from build123d import *

# Parameters (mm, degrees)
SKETCH1_W           = 355.6
SKETCH1_H           = 203.2
SKETCH1_R           = 2.413
BOSS_EXTRUDE1_DEPTH = 3.175
SKETCH2_R           = 3.81
CUT_EXTRUDE1_DEPTH  = 205.80595847


with BuildPart() as part:
    # Sketch1 → Boss-Extrude1 (new body)
    with BuildSketch(Plane(origin=(0, 0, 0), x_dir=(1, 0, 0), z_dir=(0, 1, 0))):
        Rectangle(SKETCH1_W, SKETCH1_H)
        with Locations(Location((42.8625, 74.240027739, 0), (0, 0, 270))):
            Circle(SKETCH1_R, mode=Mode.SUBTRACT)
        with Locations(Location((85.725, 0, 0), (0, 0, 270))):
            Circle(SKETCH1_R, mode=Mode.SUBTRACT)
        with Locations(Location((42.8625, -74.240027739, 0), (0, 0, 270))):
            Circle(SKETCH1_R, mode=Mode.SUBTRACT)
        with Locations(Location((-42.8625, -74.240027739, 0), (0, 0, 270))):
            Circle(SKETCH1_R, mode=Mode.SUBTRACT)
        with Locations(Location((-85.725, 0, 0), (0, 0, 270))):
            Circle(SKETCH1_R, mode=Mode.SUBTRACT)
        with Locations(Location((-42.8625, 74.240027739, 0), (0, 0, 270))):
            Circle(SKETCH1_R, mode=Mode.SUBTRACT)
    extrude(amount=BOSS_EXTRUDE1_DEPTH)

    # Sketch2 → Cut-Extrude1 (cut, through all)
    with BuildSketch(Plane(origin=(0, 3.175, 0), x_dir=(1, 0, 0), z_dir=(0, 1, 0))):
        with Locations(Location((165.1, 82.55, 0), (0, 0, 270))):
            Circle(SKETCH2_R)
        with Locations(Location((-165.1, 82.55, 0), (0, 0, 90))):
            Circle(SKETCH2_R)
        with Locations(Location((-165.1, -82.55, 0), (0, 0, 270))):
            Circle(SKETCH2_R)
        with Locations(Location((165.1, -82.55, 0), (0, 0, 90))):
            Circle(SKETCH2_R)
    extrude(amount=-CUT_EXTRUDE1_DEPTH, mode=Mode.SUBTRACT)


solid = part.part
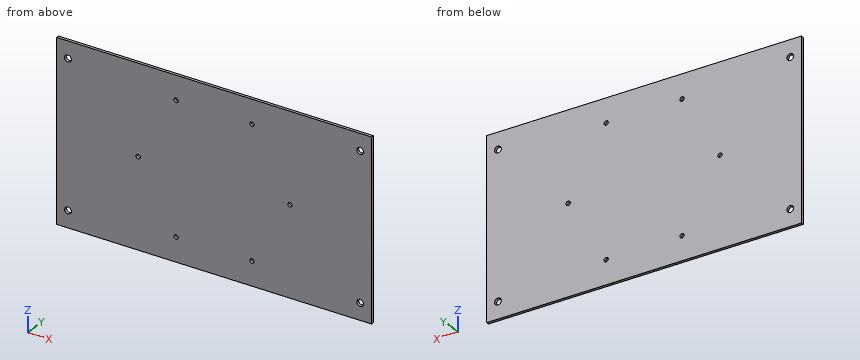
Read the model definition and answer for the solid it produces. Units are mm, in the model's axes. Give positions to 0.01 mm unless a question says otherwise; leave off trailing zeros. Write each loop counter-clockwise with the first axis right and the second up, starting at its lowest first coordinate (ties: lowest second). Pieces come first, ordered by that corner, then holes. Notation, with made-up numbers: (-30, -6) - (-25, -6) arc R23 ccw to (-25, 13) - close; hole circle Ø6 at (54.5, 11). An arc over 180 degrees is marked (long way). Return JSON: item names as keys, results as strings.
Q1. A cutting plane is placed at B-B, the plane z = 82.55. Determine the outline of the cut face in (x, y) (3 decimals).
Reply:
{"outline": "(-177.8, 0) - (-168.91, 0) - (-168.91, 3.175) - (-177.8, 3.175) - close; (-161.29, 0) - (161.29, 0) - (161.29, 3.175) - (-161.29, 3.175) - close; (168.91, 0) - (177.8, 0) - (177.8, 3.175) - (168.91, 3.175) - close"}
Q2. Consider line 1 along X through (y, z) = (1.4, 82.55); line 2 along Z through (x, y) = (42.5, 1.2); line 3 along X through (y, z) = (2.7, -73.5). Determine where each line is inside the solid, lowest interval first. Write a range as [from, to].
Reply:
{"line 1": "[-177.8, -168.91], [-161.29, 161.29], [168.91, 177.8]", "line 2": "[-101.6, -76.63], [-71.85, 71.85], [76.63, 101.6]", "line 3": "[-177.8, -45.16], [-40.57, 40.57], [45.16, 177.8]"}
Q3. A cutting plane is placed at A-A, the plane x = 165.1. Determine the outline of the cut face in (y, z) (3 decimals).
Reply:
{"outline": "(0, -101.6) - (3.175, -101.6) - (3.175, -86.36) - (0, -86.36) - close; (0, -78.74) - (3.175, -78.74) - (3.175, 78.74) - (0, 78.74) - close; (0, 86.36) - (3.175, 86.36) - (3.175, 101.6) - (0, 101.6) - close"}
